Verification items for this drawing (mm, ordinates from the low corner). A direction names the side the tool comes from. Give positions to 0.01 mm unless a question says otherwise; leave off trailing zeros. Order: outer loops, then holes, each group sorted by start corner. A loop starts at its lowest first (then second) coordinate and runs counter-clockwise, first axis right, second up. Notation, with made-up numbers: M -36.75,16 L 9.25,16 A29 ccw 9.25,48 Z; hole C 46,74 d1. An arc over 180 degrees is marked long. One line per question, with ' | ' between items. Start each with the question number.
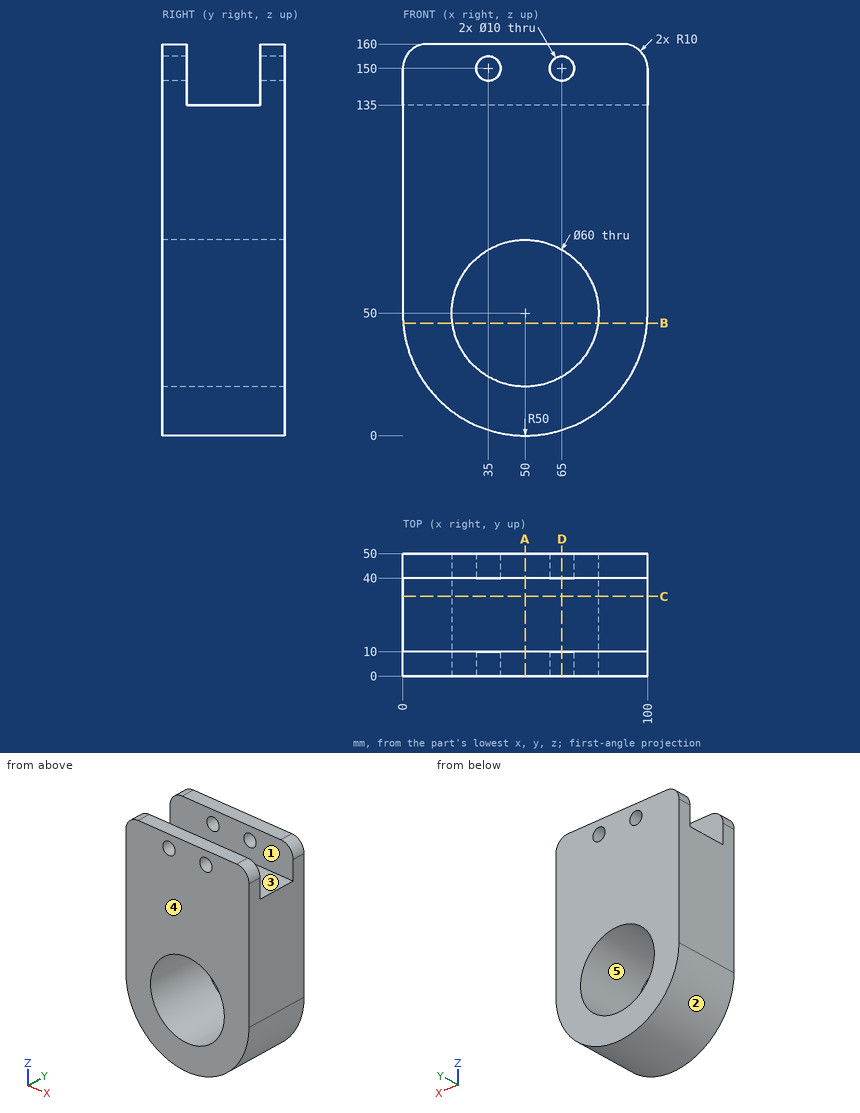
Item 1: Cross-section at C-C, the plane y = 32.5. Record the cut outline in (x, z).
Item 2: Depth check by flat-ended pin: pin 1 (1.5 mm diameter, centred on x = 72, y = 29, fed in from +Z); pin 2 (3 mm diameter, centred on x = 69.5, y = 20, fed in from -Z); pin 3 (5 mm diameter, centred on y = 7, z = 20, fed in from +X). Enter the tip coordinate at first touch or a pass-through.
Item 3: Set-up check for the marked faces 1 and 2: record each of +Z, -Z, +X, -X, +Y, -Y from which the full face is reachable in a straight line by a thin tool's end or side.
Item 4: Cross-section at D-D, the plane x = 65. Record the cut outline in (y, z).
Item 5: Cross-section at B-B, the plane z = 46. Record the cut outline in (x, y), plus the area to 3 significant figures.
Item 6: Mould release check, pull along Z, two halves, no side actions. Record for the marked faces 3, 4 and 5: released by +Z, released by -Z, zero draft, split by the parting line, or undercut.
Item 7: Cross-section at A-A, the plane x = 50. Record the cut outline in (y, z).
Item 8: Material ranges on line 1 along X through (y, z) = (42, 150); line 2 along Y through (x, z) = (91.5, 141); line 3 along Z through (x, y) = (50, 20.5), recorded low to high.
Outcome:
1) outline: M 0,50 A50 ccw 100,50 L 100,135 L 0,135 Z; hole C 50,50 d60
2) pin 1: stops at z = 135 | pin 2: stops at z = 3.35 | pin 3: stops at x = 91.76
3) face 1: +Z, +X, -X | face 2: -Z, +Y, -Y
4) outline: M 0,2.3 L 50,2.3 L 50,24.02 L 0,24.02 Z; M 0,75.98 L 50,75.98 L 50,145 L 40,145 L 40,135 L 10,135 L 10,145 L 0,145 Z; M 0,155 L 10,155 L 10,160 L 0,160 Z; M 40,155 L 50,155 L 50,160 L 40,160 Z
5) outline: M 0.16,0 L 20.27,0 L 20.27,50 L 0.16,50 Z; M 79.73,0 L 99.84,0 L 99.84,50 L 79.73,50 Z | area: 2,010 mm²
6) face 3: released by +Z | face 4: zero draft | face 5: undercut
7) outline: M 0,0 L 50,0 L 50,20 L 0,20 Z; M 0,80 L 50,80 L 50,160 L 40,160 L 40,135 L 10,135 L 10,160 L 0,160 Z
8) line 1: x = 0 to 30, 40 to 60, 70 to 100 | line 2: y = 0 to 10, 40 to 50 | line 3: z = 0 to 20, 80 to 135
